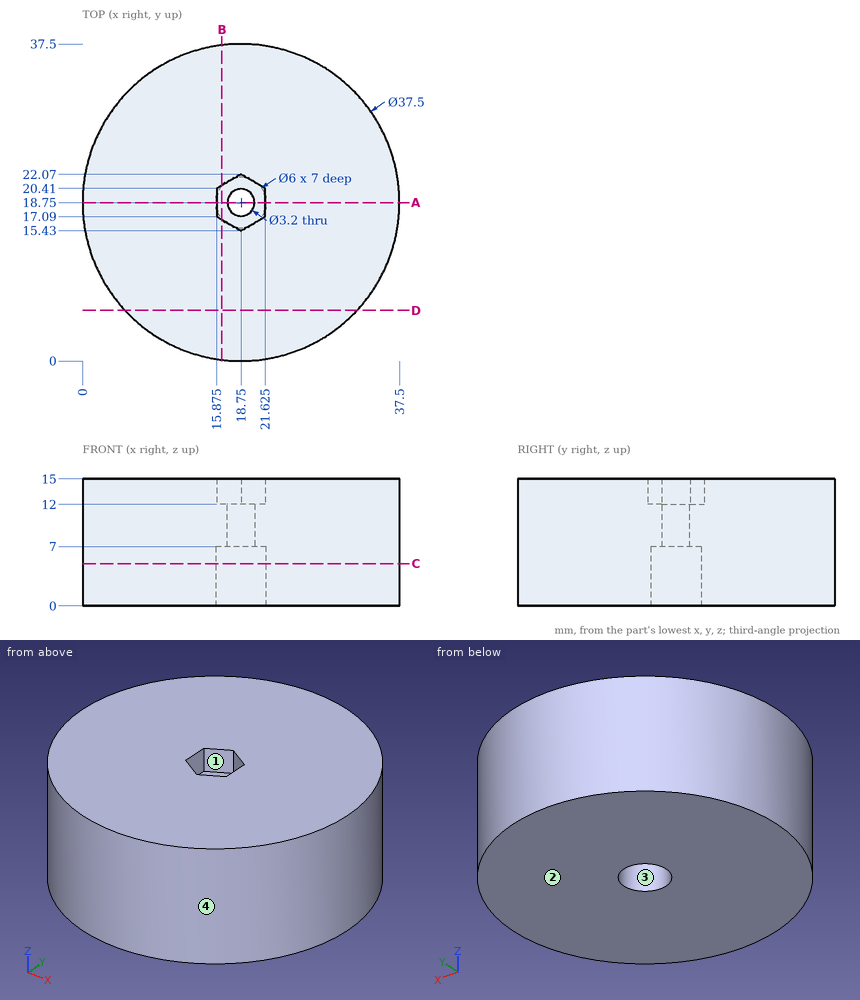
For this review, use the dimensioned drawing (mm, ordinates from the lowest corner) and the shaded views. Coordinates: 2 decimals unless noted, no trailing zeros. Write each loop counter-clockwise with the first axis right and the second up, starting at its lowest first coordinate (ties: lowest second). Pieces come first, ordered by that corner, then holes. Notation, with made-up numbers: (-28, 5) - (-5, 5) arc R34 cw to (-5, 37) - close; hole circle Ø4 at (14.25, 70). An arc over 180 degrees is marked (long way). One line per item, written item: value.
1) Add section C-C (z = 5). State the section outline as (x, y) points.
Answer sheet:
outline: circle Ø37.5 at (18.75, 18.75); hole circle Ø6 at (18.75, 18.75)
2) Add section B-B (x = 16.5). State the section outline as (y, z) points.
Answer sheet:
outline: (0.14, 0) - (16.77, 0) - (16.77, 7) - (20.73, 7) - (20.73, 0) - (37.36, 0) - (37.36, 15) - (20.77, 15) - (20.77, 12) - (16.73, 12) - (16.73, 15) - (0.14, 15) - close
3) Mouldability with a two-part tool opening along X and no side actions: class the marked faces 1, 2, 3 and 4 as +X half, -X half, draft (parallel to the pull), parting line (faces both ways), or undercut.
Answer sheet:
face 1: undercut
face 2: draft
face 3: undercut
face 4: parting line
4) Add section D-D (y = 6). State the section outline as (x, z) points, plus the area to 3 significant figures.
Answer sheet:
outline: (5, 0) - (32.5, 0) - (32.5, 15) - (5, 15) - close
area: 412 mm2
5) Add section A-A (y = 18.75). State the section outline as (x, z) points (3 decimals), plus the area to 3 significant figures.
Answer sheet:
outline: (0, 0) - (15.75, 0) - (15.75, 7) - (17.15, 7) - (17.15, 12) - (15.875, 12) - (15.875, 15) - (0, 15) - close; (20.35, 7) - (21.75, 7) - (21.75, 0) - (37.5, 0) - (37.5, 15) - (21.625, 15) - (21.625, 12) - (20.35, 12) - close
area: 487 mm2
6) To check wall thickness, follow probe 1 along Y at (x, z) = (18.75, 3); probe 2 along Y at (x, z) = (18.75, 10.15); probe 3 along X at (y, z) = (22, 11.25). State the ranges of each line that lie inside material, in increasing order.
Answer sheet:
probe 1: y = 0 to 15.75, 21.75 to 37.5
probe 2: y = 0 to 17.15, 20.35 to 37.5
probe 3: x = 0.28 to 37.22
7) Insertion check: pin 1 (3.5 mm diameter, centred on y = 18, z = 13.5, fed in from +X); pin 2 (2.5 mm diameter, centred on x = 18.75, y = 18.75, fed in from -Z); pin 3 (3 mm diameter, centred on x = 27.5, z = 9, fed in from +Y). Each pin has a flat end and moves straight along its axis. Give the tip position at first contact, or say it passes through.
Answer sheet:
pin 1: stops at x = 37.5
pin 2: passes through
pin 3: stops at y = 36.04
